Autodesk Inventor part; units mm, degrees
ref_plane "YZ Plane" through (0, 0, 0) normal (1, 0, 0) x (0, 1, 0)
ref_plane "XZ Plane" through (0, 0, 0) normal (0, 1, 0) x (-1, 0, 0)
ref_plane "XY Plane" through (0, 0, 0) normal (0, 0, 1) x (1, 0, 0)
sketch "Sketch1" plane through (0, 0, 0) normal (0, 1, 0) x (-1, 0, 0)
  line L0 (0, 0) -> (0, -117.094)
  line L1 (0, -117.094) -> (87.63, -117.094)
  line L2 (87.63, -117.094) -> (87.63, -23.622)
  line L3 (0, 0) -> (59.944, 0)
  line L4 (59.944, 0) -> (87.63, -23.622)
  circle A0 centre (43.815, -106.934) radius 3.937
  circle A1 centre (43.815, -10.16) radius 3.937
  line L5 (87.63, -117.094) -> (80.01, -117.094)
  dimension "d0" = 117.094
  dimension "d1" = 87.63
  dimension "d2" = 93.472
  dimension "d3" = 59.944
  dimension "d10" = 7.62
extrude "Extrusion3" add sketch "Sketch1" along normal blind 1.9558
sketch "Sketch2" plane through (0, 1.9558, 0) normal (0, 1, 0) x (1, 0, 0)
  line L0 (0, 117.094) -> (-87.63, 117.094)
  line L1 (-87.63, 117.094) -> (-87.63, 86.614)
  line L2 (-87.63, 117.094) -> (-87.63, 23.622)
  point P0 (0, 0)
  dimension "d19" = 30.48
sketch "Sketch3" plane through (0, 1.9558, 0) normal (0, 1, 0) x (1, 0, 0)
  line L0 (-83.82, 52.774) -> (-83.82, 84.1388)
  line L1 (-76.2, 52.774) -> (-83.82, 52.774)
  line L2 (-76.2, 84.1388) -> (-76.2, 52.774)
  line L3 (-76.2, 84.1388) -> (-83.82, 84.1388)
  circle A0 centre (-80.01, 58.9314) radius 2.0193
  circle A1 centre (-80.01, 77.9814) radius 2.0193
  point P0 (0, 0)
extrude "Extrusion4" cut sketch "Sketch3" against normal blind 25.4 contours A0 | A1
properties part number "Flywheel Motor Plate" material "Steel, Alloy"
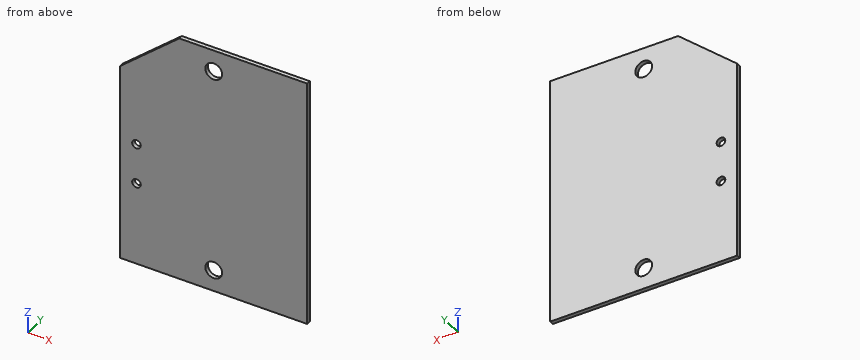
Here's how the part is built. I have some questions about the finished solid (model axes, mm). Give positions to 0.01 mm unless a question says otherwise; leave off trailing zeros. Write each loop counter-clockwise with the first axis right and the second up, starting at its lowest first coordinate (ties: lowest second). Pieces come first, ordered by that corner, then holes. Notation, with made-up numbers: (-9.5, 19.5) -> (-4.5, 19.5) arc R3 cw to (-4.5, 23.5) -> close; hole circle Ø4 at (78, 15.5). An arc over 180 degrees is marked (long way). Use one line per item in the form item = value.
1) Suppose I cut it at C-C (z = -10.16). Please give me the cut outline in (x, y), and give its area (3 significant figures).
Verdict:
outline = (-71.85, 0) -> (-47.75, 0) -> (-47.75, 1.96) -> (-71.85, 1.96) -> close; (-39.88, 0) -> (0, 0) -> (0, 1.96) -> (-39.88, 1.96) -> close
area = 125 mm2
2) Suppose I cut it at A-A (y = 0.5). Please give me the cut outline in (x, z) (3 decimals), and give its area (3 significant figures).
Verdict:
outline = (-87.63, -117.094) -> (0, -117.094) -> (0, 0) -> (-59.944, 0) -> (-87.63, -23.622) -> close; hole circle Ø4.039 at (-80.01, -77.981); hole circle Ø4.039 at (-80.01, -58.931); hole circle Ø7.874 at (-43.815, -106.934); hole circle Ø7.874 at (-43.815, -10.16)
area = 9,810 mm2
3) Suppose I cut it at D-D (x = -68). Please give me the cut outline in (y, z).
Verdict:
outline = (0, -117.09) -> (1.96, -117.09) -> (1.96, -6.87) -> (0, -6.87) -> close
4) If I drill on L1, parallel to X at y = 0.9, z = -77.5; L2, parallel to Z at x = -40.5, y = 0.75; L3, parallel to X at y = 0.2, z = -58, over which ranges is the centre line in solid material (lowest first)? Write a range as [from, to].
Verdict:
L1 = [-87.63, -81.97], [-78.05, 0]
L2 = [-117.09, -109.06], [-104.81, -12.28], [-8.04, 0]
L3 = [-87.63, -81.8], [-78.22, 0]
5) I'm going to push a flat-ended pin straight in: pin 1 (3 mm diameter, centred on x = -80.01, z = -77.98, fed in from +Y) (1 decimal). Where does the tip first touch, or does it pass through?
Verdict:
pin_1 = through
6) Suppose I cut it at B-B (x = -80.01). Please give me the cut outline in (y, z), and give its area (3 significant figures).
Verdict:
outline = (0, -117.09) -> (1.96, -117.09) -> (1.96, -80) -> (0, -80) -> close; (0, -75.96) -> (1.96, -75.96) -> (1.96, -60.95) -> (0, -60.95) -> close; (0, -56.91) -> (1.96, -56.91) -> (1.96, -17.12) -> (0, -17.12) -> close
area = 180 mm2
